Autodesk Inventor part; units mm, degrees
ref_plane "YZ Plane" through (0, 0, 0) normal (1, 0, 0) x (0, 1, 0)
ref_plane "XZ Plane" through (0, 0, 0) normal (0, 1, 0) x (-1, 0, 0)
ref_plane "XY Plane" through (0, 0, 0) normal (0, 0, 1) x (1, 0, 0)
sketch "Sketch1" plane through (0, 0, 0) normal (0, 1, 0) x (-1, 0, 0)
  line L0 (0, 0) -> (-200, 0)
  line L1 (-200, 0) -> (-200, -190)
  line L2 (-200, -190) -> (0, -190)
  line L3 (0, -190) -> (0, 0)
  line L4 (-65, 0) -> (-135, 0)
  line L5 (-135, 0) -> (-135, -5)
  line L6 (-135, -5) -> (-65, -5)
  line L7 (-65, -5) -> (-65, 0)
  line L8 (-200, -95) -> (0, -95) construction
  line L9 (-65, -190) -> (-135, -190)
  line L10 (-135, -190) -> (-135, -185)
  line L11 (-135, -185) -> (-65, -185)
  line L12 (-65, -185) -> (-65, -190)
  line L13 (-200, -215) -> (-200, -15)
  dimension "d0" = 200
  dimension "d2" = 70
  dimension "d3" = 5
  dimension "d11" = 0
  dimension "d13" = 190
extrude "Extrusion1" add sketch "Sketch1" along normal blind 5 contours L3 L2 L12 L11 L10 L1 L0 L5 L6 L7
sketch "Sketch2" plane through (0, 5, 0) normal (0, 1, 0) x (1, 0, 0)
  line L0 (0, 0) -> (65, 0)
  line L1 (135, 0) -> (200, 0)
  line L2 (65, 0) -> (65, 5)
  line L3 (0, 190) -> (0, 0)
  line L4 (0, 95) -> (200, 95)
  point P0 (95, 20)
  point P1 (105, 20)
  point P2 (95, 170)
  point P3 (105, 170)
  dimension "d22" = 20
  dimension "d23" = 10
  dimension "d24" = 20
  dimension "d25" = 30
hole "Hole1" at (95, 5, -20) at (105, 5, -20) at (95, 5, -170) at (105, 5, -170) direction (0, -1, 0) diameter 4 end through all
sketch "Sketch5" plane through (0, 5, 0) normal (0, 1, 0) x (1, 0, 0)
  line L0 (200, 0) -> (200, 190)
  line L1 (200, 190) -> (135, 190)
  point P0 (0, 0)
  point P1 (180, 90)
  point P2 (180, 100)
  dimension "d51" = 20
  dimension "d52" = 20
  dimension "d53" = 10
  dimension "d54" = 90
hole "Hole4" at (180, 5, -90) at (180, 5, -100) direction (0, -1, 0) diameter 4 end through all
properties part number "top"
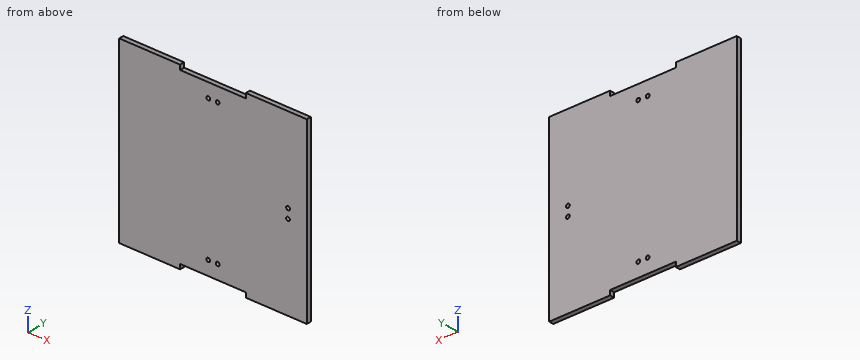
Geometry check sheet. Reference: the model listing, model coordinates, mm. Give positions to 0.01 mm unless a question says otherwise; leave off trailing zeros. Loops run counter-clockwise (first coordinate to the right, second up) from the corner with the lowest first, then second, coordinate; pieces in that order, holes last. Notation, with made-up numbers: (61, 9.5) - (111, 9.5) arc R14 ccw to (111, 33.5) - close; hole circle Ø4 at (26.25, -36.5). An arc over 180 degrees is marked (long way). Use CSV: the item, a comma, the result in double quotes. Start each with the question number.
Q1. Go/stop test with a flat-tipped pin: pin 1 Ø1.5 at (x, y) = (87.5, 1.5) entering from +Z. Record where the tip stops, or that it passes through.
Q2. Scan lines: probe 1 along Z at (x, y) = (105, 3.95); probe 2 along Z at (x, y) = (180, 4.05); probe 3 along Z at (x, y) = (117, 2.2). Record each from-to range of solid material in increasing order. Write a range as from..to.
Q3. Section check B-B, the plane x = 69. Record the cut outline in (y, z), and give its area (3 significant figures).
Q4. Section check A-A, the plane y = 3.9. Record the cut outline in (x, z), and give its area (3 significant figures).
Findings below:
1,pin 1,"stops at z = -5"
2,probe 1,"z = -185..-172, -168..-22, -18..-5"
2,probe 2,"z = -190..-102, -98..-92, -88..0"
2,probe 3,"z = -185..-5"
3,outline,"(0, -185) - (5, -185) - (5, -5) - (0, -5) - close"
3,area,"900 mm^2"
4,outline,"(0, -190) - (65, -190) - (65, -185) - (135, -185) - (135, -190) - (200, -190) - (200, 0) - (135, 0) - (135, -5) - (65, -5) - (65, 0) - (0, 0) - close; hole circle Ø4 at (95, -170); hole circle Ø4 at (95, -20); hole circle Ø4 at (105, -170); hole circle Ø4 at (105, -20); hole circle Ø4 at (180, -100); hole circle Ø4 at (180, -90)"
4,area,"37,200 mm^2"
